Print and shaded views of the part. All mm, measured from the part's lowest x, y and z. Give positions to 0.01 mm unless a question says otherwise; leave off trailing zeros. Loops run counter-clockwise (first coordinate to the right, second up) from the corner with the lowest first, then second, coordinate; pieces in that order, holes last. Notation, with made-up numbers: (53.25, 1.5) - (60.25, 1.5) arc R25 cw to (60.25, 40.5) - close; hole circle Ø7 at (80, 8.5). An arc over 180 degrees is marked (long way). Return JSON: item names as keys, results as strings.
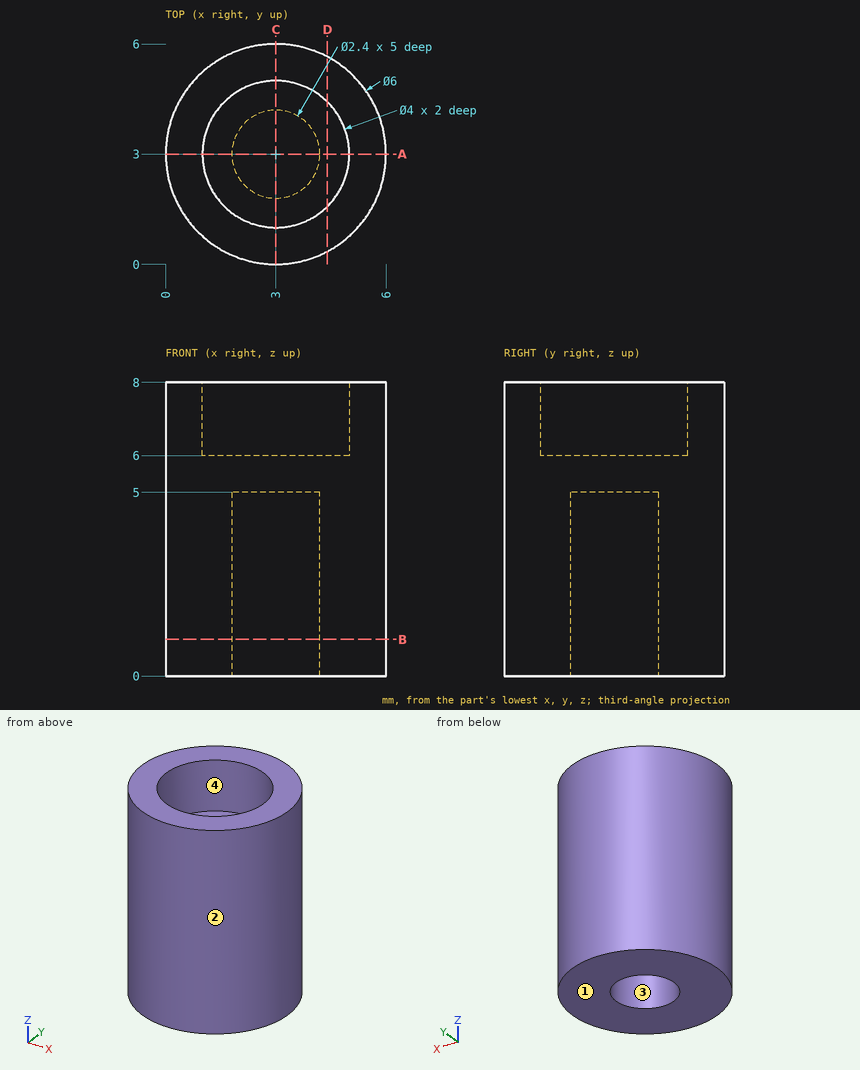
1. Pull direction X, two halves, no side cores. Call the marked faces 1, 2, 3 and 4: +X half, -X half, draft (parallel to the pull), parting line (faces both ways), or undercut.
Values follow:
{"face 1": "draft", "face 2": "parting line", "face 3": "undercut", "face 4": "undercut"}
2. Drill centre lines: probe 1 along Y at (x, z) = (3, 7.2); probe 2 along Z at (x, y) = (3.15, 1.65); probe 3 along Y at (x, z) = (3, 3.4). Where is each one in solid material? Low to high.
Values follow:
{"probe 1": "y = 0 to 1, 5 to 6", "probe 2": "z = 0 to 6", "probe 3": "y = 0 to 1.8, 4.2 to 6"}
3. Cut at A-A, the plane y = 3. Write the cut outline in (x, z), plus the area to 3 significant figures.
Values follow:
{"outline": "(0, 0) - (1.8, 0) - (1.8, 5) - (4.2, 5) - (4.2, 0) - (6, 0) - (6, 8) - (5, 8) - (5, 6) - (1, 6) - (1, 8) - (0, 8) - close", "area": "28.0 mm²"}
4. Cut at B-B, the plane z = 1. Write the cut outline in (x, y).
Values follow:
{"outline": "circle Ø6 at (3, 3); hole circle Ø2.4 at (3, 3)"}
5. Drop flat-ended pins along their axis: P1, Ø1.5, axis at y = 5, z = 6, coming from the +X side; P2, Ø0.7, axis at x = 3.5, y = 2.5, coming from the -Z side; P3, Ø1.2, axis at x = 2.5, y = 3, coming from the +Z side; P4, Ø3, axis at x = 1, y = 1, coming from the -Z side. Give the stop position or say it passes through.
Values follow:
{"P1": "stops at x = 5.73", "P2": "stops at z = 5", "P3": "stops at z = 6", "P4": "stops at z = 0"}
6. Cut at D-D, the plane x = 4.4. Write the cut outline in (y, z).
Values follow:
{"outline": "(0.35, 0) - (5.65, 0) - (5.65, 8) - (4.43, 8) - (4.43, 6) - (1.57, 6) - (1.57, 8) - (0.35, 8) - close"}
